Autodesk Inventor part; units mm, degrees
ref_plane "YZ Plane" through (0, 0, 0) normal (1, 0, 0) x (0, 1, 0)
ref_plane "XZ Plane" through (0, 0, 0) normal (0, 1, 0) x (-1, 0, 0)
ref_plane "XY Plane" through (0, 0, 0) normal (0, 0, 1) x (1, 0, 0)
sketch "Sketch1" plane through (0, 0, 0) normal (0, 0, 1) x (1, 0, 0)
  line L0 (-60, -60) -> (60, -60)
  line L1 (60, -60) -> (60, 60)
  line L2 (60, 60) -> (-60, 60)
  line L3 (-60, 60) -> (-60, -60)
  line L4 (-30, 60) -> (-24.8931, 60)
  point P0 (0, 0)
  dimension "d0" = 120
  dimension "d1" = 120
  dimension "d2" = 60
  dimension "d3" = 60
extrude "Extrusion1" add sketch "Sketch1" along normal mid plane 4
sketch "Sketch3" plane through (-60, 60, 2) normal (0, 1, 0) x (1, 0, 0)
  line L0 (120, 0) -> (0, 0)
  line L1 (0, 4) -> (120, 4)
  line L2 (0, 0) -> (12, 0)
  line L3 (12, 0) -> (12, 4)
  line L4 (12, 4) -> (0, 4)
  line L5 (0, 4) -> (0, 0)
  line L6 (0, 4) -> (0, 0)
  point P0 (60, 2)
  dimension "d17" = 0
  dimension "d18" = 12
extrude "Extrusion2" cut sketch "Sketch3" against normal blind 4
pattern_linear "side_top" count 5 spacing 24 along (1, 0, 0) of "Extrusion2"
sketch "Sketch4" plane through (-60, 56, -2) normal (-1, 0, 0) x (0, 0, 1)
  line L0 (4, 0) -> (4, -116)
  line L1 (0, -116) -> (4, -116)
  line L2 (4, -116) -> (4, -104)
  line L3 (4, -104) -> (0, -104)
  line L4 (0, -104) -> (0, -116)
  line L5 (0, -116) -> (4, -116)
  point P0 (2, -56)
  point P1 (4, -112)
  point P2 (4, -104)
  dimension "d49" = 4
  dimension "d50" = 12
  dimension "d51" = 0
  dimension "d52" = 0
extrude "Extrusion3" cut sketch "Sketch4" against normal blind 4
pattern_circular "side_bottom" count 2 over 360 about axis through (0, 0, -10) along (0, 0, 1) of "Extrusion2", "side_top"
pattern_linear "side_left" count 5 spacing 24 along (0, 1, 0) of "Extrusion3"
pattern_circular "side_right" count 2 over 360 about axis through (0, 0, -10) along (0, 0, 1) of "Extrusion3", "side_left"
sketch "Sketch6" plane through (0, 0, 2) normal (0, 0, 1) x (1, 0, 0)
  line L0 (60, -12) -> (60, 0)
  line L1 (60, 0) -> (56, 0)
  line L2 (56, 0) -> (56, 12)
  line L3 (56, 12) -> (60, 12)
  line L4 (60, 12) -> (60, 24)
  line L5 (60, 24) -> (56, 24)
  line L6 (56, 24) -> (56, 36)
  line L7 (56, 36) -> (60, 36)
  line L8 (60, 36) -> (60, 48)
  line L9 (60, 48) -> (56, 48)
  line L10 (56, 48) -> (56, 60)
  line L11 (56, 60) -> (48, 60)
  line L12 (48, 60) -> (48, 56)
  line L13 (48, 56) -> (36, 56)
  line L14 (36, 56) -> (36, 60)
  line L15 (36, 60) -> (24, 60)
  line L16 (24, 60) -> (24, 56)
  line L17 (24, 56) -> (12, 56)
  line L18 (12, 56) -> (12, 60)
  line L19 (12, 60) -> (0, 60)
  line L20 (0, 60) -> (0, 56)
  line L21 (0, 56) -> (-12, 56)
  line L22 (-12, 56) -> (-12, 60)
  line L23 (-12, 60) -> (-24, 60)
  line L24 (-24, 60) -> (-24, 56)
  line L25 (-24, 56) -> (-36, 56)
  line L26 (-36, 56) -> (-36, 60)
  line L27 (-36, 60) -> (-48, 60)
  line L28 (-48, 60) -> (-48, 56)
  line L29 (-48, 56) -> (-60, 56)
  line L30 (-60, 12) -> (-60, 0)
  line L31 (-60, 0) -> (-56, 0)
  line L32 (-56, 0) -> (-56, -12)
  line L33 (-56, -12) -> (-60, -12)
  line L34 (-60, -12) -> (-60, -24)
  line L35 (-60, -24) -> (-56, -24)
  line L36 (-56, -24) -> (-56, -36)
  line L37 (-56, -36) -> (-60, -36)
  line L38 (-60, -36) -> (-60, -48)
  line L39 (-60, -48) -> (-56, -48)
  line L40 (-56, -48) -> (-56, -60)
  line L41 (-56, -60) -> (-48, -60)
  line L42 (-48, -60) -> (-48, -56)
  line L43 (-48, -56) -> (-36, -56)
  line L44 (-36, -56) -> (-36, -60)
  line L45 (-36, -60) -> (-24, -60)
  line L46 (-24, -60) -> (-24, -56)
  line L47 (-24, -56) -> (-12, -56)
  line L48 (-12, -56) -> (-12, -60)
  line L49 (-12, -60) -> (0, -60)
  line L50 (0, -60) -> (0, -56)
  line L51 (0, -56) -> (12, -56)
  line L52 (12, -56) -> (12, -60)
  line L53 (12, -60) -> (24, -60)
  line L54 (24, -60) -> (24, -56)
  line L55 (24, -56) -> (36, -56)
  line L56 (36, -56) -> (36, -60)
  line L57 (36, -60) -> (48, -60)
  line L58 (48, -60) -> (48, -56)
  line L59 (48, -56) -> (60, -56)
  line L60 (-60.11, 60.11) -> (-35.89, 60.11)
  line L61 (-35.89, 60.11) -> (-35.89, 56.11)
  line L62 (-35.89, 56.11) -> (-24.11, 56.11)
  line L63 (-24.11, 56.11) -> (-24.11, 60.11)
  line L64 (-24.11, 60.11) -> (-11.89, 60.11)
  line L65 (-11.89, 60.11) -> (-11.89, 56.11)
  line L66 (-11.89, 56.11) -> (-0.11, 56.11)
  line L67 (-0.11, 56.11) -> (-0.11, 60.11)
  line L68 (-0.11, 60.11) -> (12.11, 60.11)
  line L69 (12.11, 60.11) -> (12.11, 56.11)
  line L70 (12.11, 56.11) -> (23.89, 56.11)
  line L71 (23.89, 56.11) -> (23.89, 60.11)
  line L72 (23.89, 60.11) -> (36.11, 60.11)
  line L73 (36.11, 60.11) -> (36.11, 56.11)
  line L74 (36.11, 56.11) -> (47.89, 56.11)
  line L75 (47.89, 56.11) -> (47.89, 60.11)
  line L76 (47.89, 60.11) -> (56.11, 60.11)
  line L77 (56.11, 60.11) -> (56.11, 48.11)
  line L78 (56.11, 48.11) -> (60.11, 48.11)
  line L79 (60.11, 48.11) -> (60.11, 35.89)
  line L80 (60.11, 35.89) -> (56.11, 35.89)
  line L81 (56.11, 35.89) -> (56.11, 24.11)
  line L82 (56.11, 24.11) -> (60.11, 24.11)
  line L83 (60.11, 24.11) -> (60.11, 11.89)
  line L84 (60.11, 11.89) -> (56.11, 11.89)
  line L85 (56.11, 11.89) -> (56.11, 0.11)
  line L86 (56.11, 0.11) -> (60.11, 0.11)
  line L87 (60.11, 0.11) -> (60.11, -22.11)
  line L88 (60.11, -22.11) -> (56.11, -22.11)
  line L89 (56.11, -22.11) -> (56.11, -33.89)
  line L90 (56.11, -33.89) -> (60.11, -33.89)
  line L91 (60.11, -33.89) -> (60.11, -24.11)
  line L92 (60.11, -24.11) -> (56.11, -24.11)
  line L93 (56.11, -24.11) -> (56.11, -35.89)
  line L94 (56.11, -35.89) -> (60.11, -35.89)
  line L95 (60.11, -35.89) -> (60.11, -68.11)
  line L96 (60.11, -68.11) -> (60.11, -68.11)
  line L97 (60.11, -68.11) -> (60.11, -72.11)
  line L98 (60.11, -72.11) -> (23.89, -72.11)
  line L99 (23.89, -72.11) -> (23.89, -68.11)
  line L100 (23.89, -68.11) -> (36.11, -68.11)
  line L101 (36.11, -68.11) -> (36.11, -72.11)
  line L102 (36.11, -72.11) -> (-0.11, -72.11)
  line L103 (-0.11, -72.11) -> (-0.11, -68.11)
  line L104 (-0.11, -68.11) -> (12.11, -68.11)
  line L105 (12.11, -68.11) -> (12.11, -72.11)
  line L106 (12.11, -72.11) -> (-24.11, -72.11)
  line L107 (-24.11, -72.11) -> (-24.11, -68.11)
  line L108 (-24.11, -68.11) -> (-11.89, -68.11)
  line L109 (-11.89, -68.11) -> (-11.89, -72.11)
  line L110 (-11.89, -72.11) -> (-48.11, -72.11)
  line L111 (-48.11, -72.11) -> (-48.11, -68.11)
  line L112 (-48.11, -68.11) -> (-35.89, -68.11)
  line L113 (-35.89, -68.11) -> (-35.89, -72.11)
  line L114 (-35.89, -72.11) -> (-68.11, -72.11)
  line L115 (-68.11, -72.11) -> (-68.11, -60.11)
  line L116 (-68.11, -60.11) -> (-72.11, -60.11)
  line L117 (-72.11, -60.11) -> (-72.11, -23.89)
  line L118 (-72.11, -23.89) -> (-68.11, -23.89)
  line L119 (-68.11, -23.89) -> (-68.11, -36.11)
  line L120 (-68.11, -36.11) -> (-72.11, -36.11)
  line L121 (-72.11, -36.11) -> (-72.11, 0.11)
  line L122 (-72.11, 0.11) -> (-68.11, 0.11)
  line L123 (-68.11, 0.11) -> (-68.11, -12.11)
  line L124 (-68.11, -12.11) -> (-72.11, -12.11)
  line L125 (-72.11, -12.11) -> (-72.11, 44.11)
  line L126 (-72.11, 44.11) -> (-68.11, 44.11)
  line L127 (-68.11, 44.11) -> (-68.11, 11.89)
  line L128 (-68.11, 11.89) -> (-72.11, 11.89)
  line L129 (-72.11, 11.89) -> (-72.11, 24.11)
  line L130 (-72.11, 24.11) -> (-68.11, 24.11)
  line L131 (-68.11, 24.11) -> (-68.11, 35.89)
  line L132 (-68.11, 35.89) -> (-72.11, 35.89)
  line L133 (-72.11, 35.89) -> (-72.11, 68.11)
  line L134 (-72.11, 68.11) -> (-60.11, 68.11)
  line L135 (-60.11, 68.11) -> (-60.11, 60.11)
  line L136 (56, -36) -> (60, -36)
  line L137 (60, -36) -> (60, -24)
  line L138 (60, -24) -> (56, -24)
  line L139 (56, -24) -> (56, -12)
  line L140 (56, -12) -> (60, -12)
  line L141 (-60, 56) -> (-60, 48)
  line L142 (-60, 48) -> (-56, 48)
  line L143 (-56, 48) -> (-56, 36)
  line L144 (-56, 36) -> (-60, 36)
  line L145 (-60, 36) -> (-60, 24)
  line L146 (-60, 24) -> (-56, 24)
  line L147 (-56, 24) -> (-56, 12)
  line L148 (-56, 12) -> (-60, 12)
  line L149 (60, -56) -> (60, -48)
  line L150 (60, -48) -> (56, -48)
  line L151 (56, -48) -> (56, -36)
  point P0 (0, 0)
  dimension "d59" = 0.11
extrude "Extrusion5" [suppressed]
sketch "Sketch7" plane through (0, 0, 2) normal (0, 0, 1) x (1, 0, 0)
  line L0 (-60.11, 68.11) -> (-72.11, 68.11)
  line L1 (-72.11, 68.11) -> (-72.11, 35.89)
  line L2 (-72.11, 35.89) -> (-68.11, 35.89)
  line L3 (-68.11, 35.89) -> (-68.11, 24.11)
  line L4 (-68.11, 24.11) -> (-72.11, 24.11)
  line L5 (-72.11, 24.11) -> (-72.11, 11.89)
  line L6 (-72.11, 11.89) -> (-68.11, 11.89)
  line L7 (-68.11, 11.89) -> (-68.11, 0.11)
  line L8 (-68.11, 0.11) -> (-72.11, 0.11)
  line L9 (-72.11, 0.11) -> (-72.11, -12.11)
  line L10 (-72.11, -12.11) -> (-68.11, -12.11)
  line L11 (-68.11, -12.11) -> (-68.11, -23.89)
  line L12 (-68.11, -23.89) -> (-72.11, -23.89)
  line L13 (-72.11, -23.89) -> (-72.11, -36.11)
  line L14 (-72.11, -36.11) -> (-68.11, -36.11)
  line L15 (-68.11, -36.11) -> (-68.11, -47.89)
  line L16 (-68.11, -47.89) -> (-72.11, -47.89)
  line L17 (-72.11, -47.89) -> (-72.11, -60.11)
  line L18 (-72.11, -60.11) -> (-68.11, -60.11)
  line L19 (-68.11, -60.11) -> (-68.11, -72.11)
  line L20 (-68.11, -72.11) -> (-35.89, -72.11)
  line L21 (-35.89, -72.11) -> (-35.89, -68.11)
  line L22 (-35.89, -68.11) -> (-24.11, -68.11)
  line L23 (-24.11, -68.11) -> (-24.11, -72.11)
  line L24 (-24.11, -72.11) -> (-11.89, -72.11)
  line L25 (-11.89, -72.11) -> (-11.89, -68.11)
  line L26 (-11.89, -68.11) -> (-0.11, -68.11)
  line L27 (-0.11, -68.11) -> (-0.11, -72.11)
  line L28 (-0.11, -72.11) -> (12.11, -72.11)
  line L29 (12.11, -72.11) -> (12.11, -68.11)
  line L30 (12.11, -68.11) -> (23.89, -68.11)
  line L31 (23.89, -68.11) -> (23.89, -72.11)
  line L32 (23.89, -72.11) -> (36.11, -72.11)
  line L33 (36.11, -72.11) -> (36.11, -68.11)
  line L34 (36.11, -68.11) -> (47.89, -68.11)
  line L35 (47.89, -68.11) -> (47.89, -72.11)
  line L36 (47.89, -72.11) -> (60.11, -72.11)
  line L37 (60.11, -72.11) -> (60.11, -68.11)
  line L38 (60.11, -68.11) -> (72.11, -68.11)
  line L39 (72.11, -68.11) -> (72.11, -35.89)
  line L40 (72.11, -35.89) -> (68.11, -35.89)
  line L41 (68.11, -35.89) -> (68.11, -24.11)
  line L42 (68.11, -24.11) -> (72.11, -24.11)
  line L43 (72.11, -24.11) -> (72.11, -11.89)
  line L44 (72.11, -11.89) -> (68.11, -11.89)
  line L45 (68.11, -11.89) -> (68.11, -0.11)
  line L46 (68.11, -0.11) -> (72.11, -0.11)
  line L47 (72.11, -0.11) -> (72.11, 12.11)
  line L48 (72.11, 12.11) -> (68.11, 12.11)
  line L49 (68.11, 12.11) -> (68.11, 23.89)
  line L50 (68.11, 23.89) -> (72.11, 23.89)
  line L51 (72.11, 23.89) -> (72.11, 36.11)
  line L52 (72.11, 36.11) -> (68.11, 36.11)
  line L53 (68.11, 36.11) -> (68.11, 47.89)
  line L54 (68.11, 47.89) -> (72.11, 47.89)
  line L55 (72.11, 47.89) -> (72.11, 60.11)
  line L56 (72.11, 60.11) -> (68.11, 60.11)
  line L57 (68.11, 60.11) -> (68.11, 72.11)
  line L58 (68.11, 72.11) -> (35.89, 72.11)
  line L59 (35.89, 72.11) -> (35.89, 68.11)
  line L60 (35.89, 68.11) -> (24.11, 68.11)
  line L61 (24.11, 68.11) -> (24.11, 72.11)
  line L62 (24.11, 72.11) -> (11.89, 72.11)
  line L63 (11.89, 72.11) -> (11.89, 68.11)
  line L64 (11.89, 68.11) -> (0.11, 68.11)
  line L65 (0.11, 68.11) -> (0.11, 72.11)
  line L66 (0.11, 72.11) -> (-12.11, 72.11)
  line L67 (-12.11, 72.11) -> (-12.11, 68.11)
  line L68 (-12.11, 68.11) -> (-23.89, 68.11)
  line L69 (-23.89, 68.11) -> (-23.89, 72.11)
  line L70 (-23.89, 72.11) -> (-36.11, 72.11)
  line L71 (-36.11, 72.11) -> (-36.11, 68.11)
  line L72 (-36.11, 68.11) -> (-47.89, 68.11)
  line L73 (-47.89, 68.11) -> (-47.89, 72.11)
  line L74 (-47.89, 72.11) -> (-60.11, 72.11)
  line L75 (-60.11, 72.11) -> (-60.11, 68.11)
  point P0 (0, 0)
equation "\"d0\" = width"
equation "\"d1\" = height"
equation "\"d4\" = thickness"
equation "\"d18\" = finger"
equation "\"d19\" = thickness"
equation "\"d23\" = 2 * finger"
equation "\"d49\" = thickness"
equation "\"d50\" = finger"
equation "\"d28\" = thickness"
equation "\"d55\" = 2 * finger"
equation "\"d59\" = 0.5 * kerf"
equation "\"d60\" = thickness"
equation "\"width\" = 120"
equation "\"height\" = 120"
equation "\"thickness\" = 4"
equation "\"finger\" = 3 * thickness"
equation "\"kerf\" = 0.22"
properties part number "Lukt_hlidarplata"
Build history of the part. All positions in model axes, mm. A direction names the side the tool comes from. Coordinates: 2 decimals unless noted, no trailing zeros. Write each loop counter-clockwise with the first axis right and the second up, starting at its lowest first coordinate (ties: lowest second). Pieces come first, ordered by that corner, then holes. Notation, with made-up numbers: (69.5, 47.25) -> (109.5, 47.25) arc R15 ccw to (109.5, 61.25) -> close; hole circle Ø6 at (53.5, 2). An arc over 180 degrees is marked (long way). Use CSV: the item, a comma, the result in double quotes. Start each with the question number.
Q1. Flat gauge pins, fed straight in: pin 1 Ø1 at (y, z) = (7, 0.5) entering from +X; pin 2 Ø1.2 at (x, z) = (-57, 0) entering from -Y; pin 3 Ø2 at (y, z) = (18, -0.5) entering from -X. Where does each tip first touch, or does it go through?
Q2. Drill centre lines: probe 1 along X at (y, z) = (-53, -1.6); probe 2 along Y at (x, z) = (-4.5, 0.4). Where is each one in solid material? Low to high.
Q3. Cut at A-A, the plane x = -29.5. List the corners of the cut face in (y, z), then the cut area to 3 significant figures.
Q4. 3-axis set-ups, long thin cutter, end or side, ignore diameter. For faces 1 (the flat face through (-58, -12, 0)), 2 (the flat face through (-56, -54, 0)), 3 (the flat face through (56, -18, 0)), 4 (the flat face through (30, -56, 0)): which of +Z, -Z, +X, -X, +Y, -Y reach the whole face in a straight line?
Q5. Pull direction X, two halves, no side cores. Call faces 5 (the flat face through (-60, 6, 0)), 6 (the flat face through (48, -58, 0)), 7 (the flat face through (0, -58, 0)): released by +X, released by -X, zero draft, split by the parting line, or undercut.
Checked values:
1,pin 1,"stops at x = 56"
1,pin 2,"stops at y = -48"
1,pin 3,"stops at x = -56"
2,probe 1,"x = -56 to 60"
2,probe 2,"y = -60 to 56"
3,outline,"(-60, -2) -> (56, -2) -> (56, 2) -> (-60, 2) -> close"
3,area,"464 mm²"
4,face 1,"+Z, -Z, -X"
4,face 2,"+Z, -Z, -X, -Y"
4,face 3,"+Z, -Z, +X"
4,face 4,"+Z, -Z, -Y"
5,face 5,"released by -X"
5,face 6,"released by +X"
5,face 7,"undercut"
